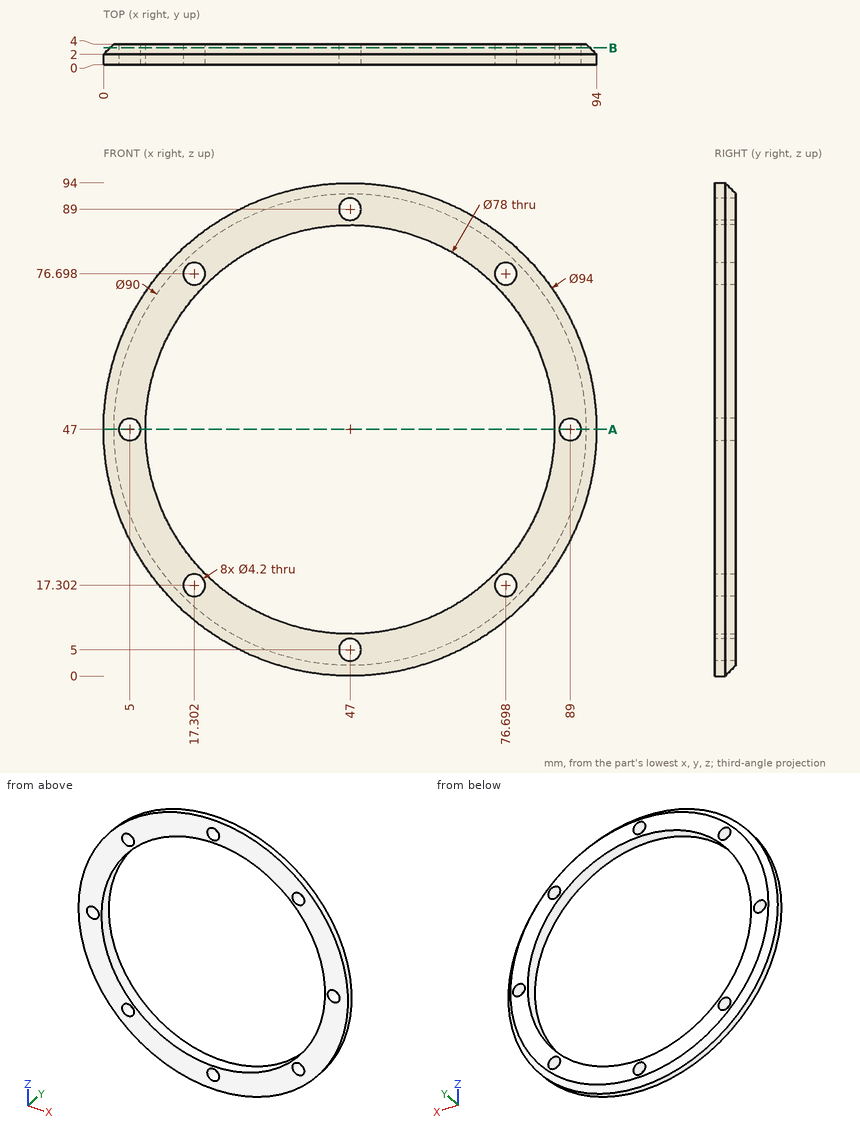
Part print with two shaded views. Sizes in mm from the minimum x, y, z corner. Coordinates: 2 decimals unless noted, no trailing zeros. Write each loop counter-clockwise with the first axis right and the second up, starting at its lowest first coordinate (ties: lowest second). Pieces come first, ordered by that corner, then holes. Notation, with made-up numbers: M -18,33 L 37,33 A26 ccw 37,62 Z; hole C 2,3 d8. An arc over 180 degrees is marked long. Return JSON: item names as keys, results as strings.
Item 1: Drop flat-ended pins along their axis: pin 1 Ø2 at (x, y) = (59.5, 1.5) entering from +Z; pin 2 Ø1 at (y, z) = (3, 78) entering from +X (1 decimal); pin 3 Ø1.5 at (x, y) = (33.5, 2) entering from -Z. Give the stop position or say it passes through.
Findings below:
{"pin 1": "stops at z = 92.57", "pin 2": "stops at x = 81.8", "pin 3": "stops at z = 1.76"}
Item 2: Slice it at B-B, the plane y = 3.25. State how many separate pieces and enclosed holes the cut face has, and give its area (3 significant figures).
Findings below:
{"separate pieces": "1", "enclosed holes": "9", "area": "1,690 mm2"}
Item 3: Slice it at A-A, the plane z = 47. Write the cut outline in (x, y), and give its area (3 significant figures).
Findings below:
{"outline": "M 0,0 L 2.9,0 L 2.9,4 L 2,4 L 0,2 Z; M 7.1,0 L 8,0 L 8,4 L 7.1,4 Z; M 86,0 L 86.9,0 L 86.9,4 L 86,4 Z; M 91.1,0 L 94,0 L 94,2 L 92,4 L 91.1,4 Z", "area": "26.4 mm2"}
Item 4: Probe line 1 (Z direction, x = 47, y = 0.9); line 2 (X direction, y = 0.75, z = 77) (1 decimal); line 3 (X direction, y = 3.55, z = 77) (1 decimal). List the from-to ranges inside material, lowest first. Write a range as from..to.
Findings below:
{"line 1": "z = 0..2.9, 7.1..8, 86..86.9, 91.1..94", "line 2": "x = 10.8..15.2, 19.4..22.1, 71.9..74.6, 78.8..83.2", "line 3": "x = 12.9..15.2, 19.4..22.1, 71.9..74.6, 78.8..81.1"}
